from build123d import *

# Parameters (mm, degrees)
SKETCH1_W            = 22.5
SKETCH1_H            = 7.5
BOSS_EXTRUDE1_DEPTH  = 16
SKETCH2_R            = 3.25
CUT_EXTRUDE1_DEPTH   = 29.609439002
CUT_SWEEP1_START     = -5.5
CUT_SWEEP1_DEPTH     = 5.5
M8_CLEARANCE_HOLE1_D = 9
FILLET1_R            = 7.5


# Read off the part's stored shape, not the designer's step: Cut-Sweep1
with BuildPart() as part:
    # Sketch1 → Boss-Extrude1 (new body)
    with BuildSketch(Plane(origin=(0, 0, 0), x_dir=(1, 0, 0), z_dir=(0, 1, 0))):
        with Locations((11.25, 3.75)):
            Rectangle(SKETCH1_W, SKETCH1_H)
    extrude(amount=BOSS_EXTRUDE1_DEPTH)

    # Sketch2 → Cut-Extrude1 (cut, through all)
    with BuildSketch(Plane.XY):
        with Locations((0, 8)):
            Circle(SKETCH2_R)
    extrude(amount=-CUT_EXTRUDE1_DEPTH, mode=Mode.SUBTRACT)

    # Cut-Sweep1 outline → Cut-Sweep1 (cut)
    with BuildSketch(Plane.XY.offset(CUT_SWEEP1_START)):
        with BuildLine():
            Line((0, 3.249930627), (0, 1.249434771))
            add(Edge.make_bspline(
                [(0, 1.249434771), (0.149995203, 1.25004033), (0.30688463, 1.254968997), (1.093425095, 1.310005949), (1.780407601, 1.443456641), (3.214381438, 2.014530663), (3.966417034, 2.456250234), (5.342873723, 3.766883929), (5.956791785, 4.632955322), (6.725554437, 6.74015649), (6.857452883, 7.944240799), (6.449506923, 10.330582428), (5.919057461, 11.44506695), (4.432172795, 13.221075917), (3.517243631, 13.845944042), (1.687026948, 14.610603142), (0.802645598, 14.750006388), (0, 14.75)],
                knots=[0.087190704, 0.087190704, 0.087190704, 0.087190704, 0.118471805, 0.118471805, 0.23694361, 0.23694361, 0.355415415, 0.355415415, 0.47388722, 0.47388722, 0.592359026, 0.592359026, 0.710830831, 0.710830831, 0.829302636, 0.829302636, 0.947774441, 0.947774441, 0.947774441, 0.947774441], degree=3))
            Line((0, 14.75), (0, 12.75))
            add(Edge.make_bspline(
                [(0, 3.249930627), (0.109137324, 3.250243145), (0.218715414, 3.253689733), (0.769523599, 3.292231999), (1.251212609, 3.385472533), (2.263638937, 3.788666681), (2.793426306, 4.100980011), (3.757556078, 5.019003289), (4.195566344, 5.640878482), (4.729047664, 7.103163163), (4.82290714, 7.976601279), (4.54124976, 9.62420025), (4.15661699, 10.434633992), (3.127582079, 11.66376284), (2.470103133, 12.115899669), (1.192161348, 12.64981872), (0.547543704, 12.750002903), (0, 12.75)],
                knots=[0.087942654, 0.087942654, 0.087942654, 0.087942654, 0.118471805, 0.118471805, 0.23694361, 0.23694361, 0.355415415, 0.355415415, 0.47388722, 0.47388722, 0.592359026, 0.592359026, 0.710830831, 0.710830831, 0.829302636, 0.829302636, 0.947774441, 0.947774441, 0.947774441, 0.947774441], degree=3))
        make_face()
    extrude(amount=CUT_SWEEP1_DEPTH, mode=Mode.SUBTRACT)

    # Mirror1: part across plane


with BuildPart() as part_1:
    add(part.part)
    add(part.part.mirror(Plane(origin=(0, 16, 0), x_dir=(1, 0, 0), z_dir=(0, 0, -1))))

    # M8 Clearance Hole1 (through all)
    with Locations(Plane(origin=(0, 16, 0), x_dir=(1, 0, 0), z_dir=(0, 1, 0))):
        with Locations((15, 0)):
            Hole(M8_CLEARANCE_HOLE1_D / 2)

    # Fillet1
    fillet1_edges = [part_1.edges().sort_by_distance(p)[0] for p in [
        (22.5, 8, -7.5),
        (22.5, 8, 7.5),
    ]]
    fillet(fillet1_edges, radius=FILLET1_R - 0.0001)  # a hair under: the kernel refuses the full size


solid = part_1.part
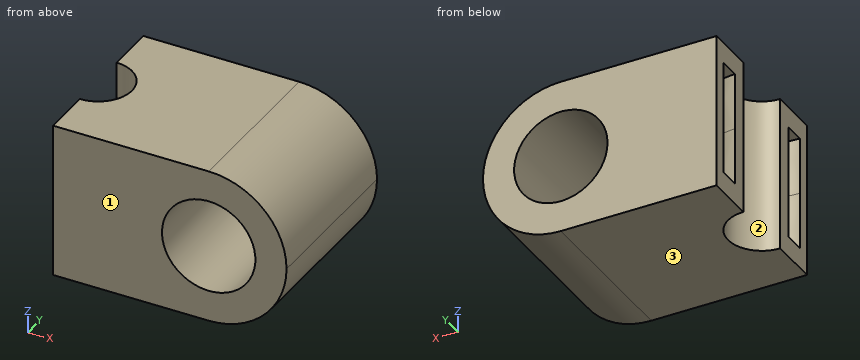
The listing builds one solid part. Answer for the finished solid, in the listing's coordinates (mm). Face numbers are marked on the shaded views. Give positions to 0.01 mm unless a question says otherwise; leave off trailing zeros. Order: outer loops, then holes, each group sorted by start corner. A loop starts at its lowest first (then second) coordinate and runs counter-clockwise, first axis right, second up. Notation, with made-up numbers: (28.25, 75.5) -> (71.25, 75.5) arc R20 cw to (71.25, 96.5) -> close; hole circle Ø8 at (77, 57). An arc over 180 degrees is marked (long way). Put each result on its own line as item: value.
Item 1: Given P1, Ø1.5, axis at x = 18, y = 14, coming from the -Z side, flat-ended and moving along its own axis, determine where the tip first touches the part or whether it passes through.
Established:
P1: stops at z = -7.15
Item 2: A cutting plane is placed at B-B on z = 2.5. Count the separate pieces of the cut face and the enclosed holes in it, plus the area to 3 significant figures.
Established:
separate pieces: 3
enclosed holes: 0
area: 181 mm^2
Item 3: A cutting plane is placed at C-C on x = 17.5. Give the vertices of the cut face in (y, z).
Established:
outline: (0, -7.07) -> (16, -7.07) -> (16, -3.74) -> (0, -3.74) -> close; (0, 3.74) -> (16, 3.74) -> (16, 7.07) -> (0, 7.07) -> close
Item 4: A cutting plane is placed at A-A on x = 13.25. Give the vertices of the cut face in (y, z).
Established:
outline: (0, -7.5) -> (16, -7.5) -> (16, -4.15) -> (0, -4.15) -> close; (0, 4.15) -> (16, 4.15) -> (16, 7.5) -> (0, 7.5) -> close
Item 5: Straight lines are drawn through the part: line 1 (Z direction, x = 15, y = 9); line 2 (Y direction, x = 4, z = -5.25); line 3 (X direction, y = 9, z = -1.5). For each, find the intervals that lie inside material, in ascending order.
Established:
line 1: z = -7.5 to -4.5, 4.5 to 7.5
line 2: y = 0 to 2.56, 5.44 to 10.56, 13.44 to 16
line 3: x = 3.09 to 4.64, 6.68 to 10.76, 19.24 to 22.35
Item 6: For a pull along Y with two mould halves and no side action, classify the marked faces 1, 2 and 3 as released by +Y, released by -Y, zero draft, split by the parting line, or undercut.
Established:
face 1: released by -Y
face 2: undercut
face 3: zero draft
